Source: CAD feature listing. Evaluate the final solid. Frame: model axes, mm. A direction names the side the tool comes from. Give positions to 0.01 mm unless a question says otherwise; leave off trailing zeros. Order: outer loops, then holes, each group sorted by start corner. A loop starts at its lowest first (then second) coordinate and runs counter-clockwise, first axis right, second up.
from build123d import *

# Parameters (mm, degrees)
BOSS_EXTRUDE1_DEPTH = 88.9
SKETCH2_R           = 2.54
SKETCH2_R_2         = 2.922857965
CUT_EXTRUDE1_DEPTH  = 88.9
SKETCH3_R           = 3.175
CUT_EXTRUDE2_DEPTH  = 88.9


with BuildPart() as part:
    # Sketch1 → Boss-Extrude1 (new body)
    with BuildSketch(Plane(origin=(0, 0, 0), x_dir=(1, 0, 0), z_dir=(0, 1, 0))):
        Polygon((0, 25.4), (0, 0), (25.4, 0), (25.4, 1.5875), (1.5875, 1.5875), (1.5875, 25.4), align=None)
    extrude(amount=BOSS_EXTRUDE1_DEPTH)

    # Sketch2 → Cut-Extrude1 (cut)
    with BuildSketch(Plane(origin=(0, 0, -1.5875), x_dir=(-1, 0, 0), z_dir=(0, 0, -1))):
        with Locations((-13.612947448, 12.7)):
            Circle(SKETCH2_R)
        with Locations((-13.612947448, 38.1)):
            Circle(SKETCH2_R_2)
    extrude(amount=-CUT_EXTRUDE1_DEPTH, mode=Mode.SUBTRACT)

    # Sketch3 → Cut-Extrude2 (cut)
    with BuildSketch(Plane(origin=(1.5875, 0, 0), x_dir=(0, 0, -1), z_dir=(1, 0, 0))):
        with Locations((12.7, 76.2)):
            Circle(SKETCH3_R)
    extrude(amount=-CUT_EXTRUDE2_DEPTH, mode=Mode.SUBTRACT)


solid = part.part
1) Section query A-A on y = 12.7. Output: boundary loops of the cut face in (x, z), and give its area (3 significant figures).
Checks:
outline: (0, -25.4) - (1.59, -25.4) - (1.59, -1.59) - (11.07, -1.59) - (11.07, 0) - (0, 0) - close; (16.15, -1.59) - (25.4, -1.59) - (25.4, 0) - (16.15, 0) - close
area: 70.1 mm2
2) First-contact query: pin 1 Ø12 at (y, z) = (74, -19) entering from +X; pin 2 Ø5 at (x, y) = (5, 23) entering from -Z. Flat tips, straight axial feed; report the tip coordinate or a pass-through.
Checks:
pin 1: stops at x = 1.59
pin 2: stops at z = -1.59
3) Section query B-B on z = -12.7. Output: boundary loops of the cut face in (x, y) (1 decimal).
Checks:
outline: (0, 0) - (1.6, 0) - (1.6, 73) - (0, 73) - close; (0, 79.4) - (1.6, 79.4) - (1.6, 88.9) - (0, 88.9) - close
4) Section query C-C on y = 38.1. Output: boundary loops of the cut face in (x, z).
Checks:
outline: (0, -25.4) - (1.59, -25.4) - (1.59, -1.59) - (10.69, -1.59) - (10.69, 0) - (0, 0) - close; (16.54, -1.59) - (25.4, -1.59) - (25.4, 0) - (16.54, 0) - close
5) Ray query, L1, parallel to X at y = 55, z = -7.25; L2, parallel to Z at x = 12.5, y = 27. Return the intervals inside material, ascending.
Checks:
L1: x = 0 to 1.59
L2: z = -1.59 to 0
6) Pull-direction query (Y, two-part tool) for faces 1 (the face through (15.5, 14.4, -0.8)), 2 (the face through (1, 88.9, -7)), 3 (the face through (14.247, 35.247, -0.805)), 4 (the face through (25.4, 44, -1)); classes: +Y half, -Y half, draft (parallel to the pull), parting line (faces both ways), or undercut.
Checks:
face 1: undercut
face 2: +Y half
face 3: undercut
face 4: draft
7) Reachability of faces 5 (the face through (1, 44, -25.4)), 6 (the face through (14, 44, -1.588)) from +Z, -Z, +X, -X, +Y, -Y: full face, straight path, thin tool, end or side. Return the list, or none.
Checks:
face 5: -Z, +X, -X, +Y, -Y
face 6: -Z, +X, +Y, -Y
8) Section query D-D on x = 6.75. Output: boundary loops of the cut face in (y, z).
Checks:
outline: (0, -1.59) - (88.9, -1.59) - (88.9, 0) - (0, 0) - close
